Could you check a few things on this model? Use its own coordinates, in mm. A direction names the side the tool comes from. Give positions to 0.01 mm unless a question says otherwise; leave off trailing zeros. Write each loop counter-clockwise with the first axis right and the second up, starting at its lowest first coordinate (ties: lowest second). Pieces come first, ordered by that corner, then holes. Notation, with made-up numbers: (-22, -3) - (-16, -3) arc R27 ccw to (-16, 25) - close; hole circle Ø2 at (59.5, 86.5). An arc over 180 degrees is marked (long way). Answer in a Markdown table with one row per item.
from build123d import *

# Parameters (mm, degrees)
EXTRUDE_1_DEPTH          = 35
SKETCH_3_W               = 25
SKETCH_3_H               = 19
CUT_EXTRUDE_1_DEPTH      = 181.230887126
SKETCH_4_W               = 25
SKETCH_4_H               = 12.5
CUT_EXTRUDE_2_DEPTH      = 13.5
SKETCH_5_W               = 25
SKETCH_5_H               = 32
CUT_EXTRUDE_3_DEPTH      = 10
FILLET_1_R               = 3
FILLET_2_R               = 2
CUT_EXTRUDE_4_DEPTH      = 191.354670013
CUT_EXTRUDE_4_DEPTH_BACK = 191.354670013
SKETCH_6_R               = 1.5
CUT_EXTRUDE_5_DEPTH      = 189.803867534
CUT_EXTRUDE_5_DEPTH_BACK = 189.803867534
SKETCH_7_R               = 1.5
SKETCH_8_W               = 13.5
SKETCH_8_H               = 44
SKETCH_8_W_2             = 10
SKETCH_8_H_2             = 32
CUT_EXTRUDE_6_DEPTH      = 193.807936548
CUT_EXTRUDE_7_DEPTH      = 10
CUT_EXTRUDE_8_DEPTH      = 18
FILLET_3_R               = 2
SKETCH_11_W              = 10
SKETCH_11_H              = 32
EXTRUDE_2_DEPTH          = 5
CUT_EXTRUDE_10_DEPTH     = 5


with BuildPart() as part:
    # 草图1 → 凸台-拉伸1 (new body)
    with BuildSketch(Plane.XY):
        with BuildLine():
            Line((42.832374142, 47.594424801), (27.642544089, 62.784254855))
            ThreePointArc((27.642544089, 62.784254855), (27.40357385, 62.943929664), (27.121689234, 63))
            Line((27.121689234, 63), (14.544073956, 63))
            Line((14.544073956, 63), (14.544073956, 3))
            Line((14.544073956, 3), (27.121689234, 3))
            ThreePointArc((27.121689234, 3), (27.40357385, 3.056070336), (27.642544089, 3.215745145))
            Line((27.642544089, 3.215745145), (42.832374142, 18.405575199))
            ThreePointArc((42.832374142, 18.405575199), (44.044614428, 19.215568261), (45.474549341, 19.5))
            Line((45.474549341, 19.5), (159.121689234, 19.5))
            ThreePointArc((159.121689234, 19.5), (160.551624147, 19.215568261), (161.763864432, 18.405575199))
            Line((161.763864432, 18.405575199), (170.453694486, 9.715745145))
            ThreePointArc((170.453694486, 9.715745145), (170.692664725, 9.556070336), (170.974549341, 9.5))
            Line((170.974549341, 9.5), (179.738422147, 9.5))
            Line((179.738422147, 9.5), (179.738422147, 56.5))
            Line((179.738422147, 56.5), (170.974549341, 56.5))
            ThreePointArc((170.974549341, 56.5), (170.692664725, 56.443929664), (170.453694486, 56.284254855))
            Line((170.453694486, 56.284254855), (161.763864432, 47.594424801))
            ThreePointArc((161.763864432, 47.594424801), (160.551624147, 46.784431739), (159.121689234, 46.5))
            Line((159.121689234, 46.5), (45.474549341, 46.5))
            ThreePointArc((45.474549341, 46.5), (44.044614428, 46.784431739), (42.832374142, 47.594424801))
        make_face()
    extrude(amount=EXTRUDE_1_DEPTH)

    # 草图3 → 切除-拉伸1 (cut, through all)
    with BuildSketch(Plane.ZY.offset(-14.544073956)):
        with Locations((17.5, 33)):
            Rectangle(SKETCH_3_W, SKETCH_3_H)
    extrude(amount=-CUT_EXTRUDE_1_DEPTH, mode=Mode.SUBTRACT)

    # 草图4 → 切除-拉伸2 (cut)
    with BuildSketch(Plane.ZY.offset(-14.544073956)):
        with Locations((17.5, 48.75)):
            Rectangle(SKETCH_4_W, SKETCH_4_H)
        with Locations((17.5, 17.25)):
            Rectangle(SKETCH_4_W, SKETCH_4_H)
    extrude(amount=-CUT_EXTRUDE_2_DEPTH, mode=Mode.SUBTRACT)

    # 草图5 → 切除-拉伸3 (cut)
    with BuildSketch(Plane(origin=(179.738422147, 0, 0), x_dir=(0, 0, -1), z_dir=(1, 0, 0))):
        with Locations((-17.5, 33)):
            Rectangle(SKETCH_5_W, SKETCH_5_H)
    extrude(amount=-CUT_EXTRUDE_3_DEPTH, mode=Mode.SUBTRACT)

    # 圆角1
    fillet_1_edges = [part.edges().sort_by_distance(p)[0] for p in [
        (169.738422147, 23.5, 17.5),
        (169.738422147, 42.5, 17.5),
        (28.044073956, 42.5, 17.5),
        (28.044073956, 23.5, 17.5),
    ]]
    fillet(fillet_1_edges, radius=FILLET_1_R)

    # 圆角2
    fillet_2_edges = [part.edges().sort_by_distance(p)[0] for p in [
        (179.738422147, 56.5, 17.5),
        (179.738422147, 9.5, 17.5),
        (14.544073956, 3, 17.5),
        (14.544073956, 63, 17.5),
    ]]
    fillet(fillet_2_edges, radius=FILLET_2_R)

    # 草图6 → 切除-拉伸4 (cut, two sides: drawn at the far end of the back side and taken through both)
    with BuildSketch(Plane.XZ.offset(-55).offset(-CUT_EXTRUDE_4_DEPTH_BACK)):
        with Locations((23.121689234, 25)):
            Circle(SKETCH_6_R)
        with Locations((23.121689234, 10)):
            Circle(SKETCH_6_R)
    extrude(amount=CUT_EXTRUDE_4_DEPTH + CUT_EXTRUDE_4_DEPTH_BACK, mode=Mode.SUBTRACT)

    # 草图7 → 切除-拉伸5 (cut, two sides: drawn at the far end of the back side and taken through both)
    with BuildSketch(Plane.XZ.offset(-49).offset(-CUT_EXTRUDE_5_DEPTH_BACK)):
        with Locations(Location((174.974549341, 25, 0), (0, 0, 270))):
            Circle(SKETCH_7_R)
        with Locations(Location((174.974549341, 10, 0), (0, 0, 270))):
            Circle(SKETCH_7_R)
    extrude(amount=CUT_EXTRUDE_5_DEPTH + CUT_EXTRUDE_5_DEPTH_BACK, mode=Mode.SUBTRACT)

    # 草图8 → 切除-拉伸6 (cut, through all)
    with BuildSketch(Plane.XY.offset(5)):
        with Locations((21.294073956, 33)):
            Rectangle(SKETCH_8_W, SKETCH_8_H)
        with Locations((174.738422147, 33)):
            Rectangle(SKETCH_8_W_2, SKETCH_8_H_2)
    extrude(amount=-CUT_EXTRUDE_6_DEPTH, mode=Mode.SUBTRACT)

    # 草图9 → 切除-拉伸7 (cut)
    with BuildSketch(Plane(origin=(0, 0, 30), x_dir=(-1, 0, 0), z_dir=(0, 0, -1))):
        Polygon((-169.738422147, 49), (-179.738422147, 49), (-179.738422147, 17), (-169.738422147, 17), (-169.738422147, 20.5), (-169.738422147, 45.5), align=None)
    extrude(amount=-CUT_EXTRUDE_7_DEPTH, mode=Mode.SUBTRACT)

    # 草图10 → 切除-拉伸8 (cut)
    with BuildSketch(Plane.XY.offset(35)):
        with BuildLine():
            Line((169.738422147, 55.568982516), (169.738422147, 49))
            Line((169.738422147, 49), (179.738422147, 49))
            Line((179.738422147, 49), (179.738422147, 54.5))
            ThreePointArc((179.738422147, 54.5), (179.15263571, 55.914213562), (177.738422147, 56.5))
            Line((177.738422147, 56.5), (170.974549341, 56.5))
            ThreePointArc((170.974549341, 56.5), (170.692664725, 56.443929664), (170.453694486, 56.284254855))
            Line((170.453694486, 56.284254855), (169.738422147, 55.568982516))
        make_face()
    extrude(amount=-CUT_EXTRUDE_8_DEPTH, mode=Mode.SUBTRACT)

    # 圆角3
    fillet_3_edges = [part.edges().sort_by_distance(p)[0] for p in [
        (169.738422147, 55.568982516, 26),
    ]]
    fillet(fillet_3_edges, radius=FILLET_3_R)

    # 草图11 → 凸台-拉伸2 (add)
    with BuildSketch(Plane(origin=(0, 0, 0), x_dir=(-1, 0, 0), z_dir=(0, 0, -1))):
        with Locations((-174.738422147, 33)):
            Rectangle(SKETCH_11_W, SKETCH_11_H)
    extrude(amount=-EXTRUDE_2_DEPTH)

    # 草图12 → 切除-拉伸10 (cut)
    with BuildSketch(Plane(origin=(0, 0, 30), x_dir=(-1, 0, 0), z_dir=(0, 0, -1))):
        with BuildLine():
            Line((-166.738422147, 23.5), (-166.738422147, 42.5))
            ThreePointArc((-166.738422147, 42.5), (-168.859742491, 43.378679656), (-169.738422147, 45.5))
            Line((-169.738422147, 45.5), (-169.738422147, 20.5))
            ThreePointArc((-169.738422147, 20.5), (-168.859742491, 22.621320344), (-166.738422147, 23.5))
        make_face()
    extrude(amount=-CUT_EXTRUDE_10_DEPTH, mode=Mode.SUBTRACT)


solid = part.part
1) Will these pins go through, and if not, where does the flat tip stop? P1, Ø12.5, axis at x = 125, z = 18.5, coming from the +Y side; P2, Ø2, axis at x = 48.5, z = 29.5, coming from the -Y side; P3, Ø4, axis at y = 34, z = 28.5, coming from the +X side.
Check values:
| item | result |
|---|---|
| P1 | stops at y = 46.5 |
| P2 | stops at y = 19.5 |
| P3 | stops at x = 166.74 |
2) If I drill on line 1 (Y direction, x = 76, z = 21); line 2 (Z direction, x = 92.5, y = 36.5); line 3 (X direction, y = 58.25, z = 10), over which ranges is the centre line in solid material (lowest first)?
Check values:
| item | result |
|---|---|
| line 1 | y = 19.5 to 23.5, 42.5 to 46.5 |
| line 2 | z = 0 to 5, 30 to 35 |
| line 3 | x = 14.54 to 21.62, 24.62 to 32.18 |
3) Imagine slicing it at A-A (y = 39.5). List the corners of the cut face in (x, z) for me, then the cut area to 3 significant figures.
Check values:
| item | result |
|---|---|
| outline | (14.54, 30) - (166.74, 30) - (166.74, 35) - (14.54, 35) - close; (28.04, 0) - (179.74, 0) - (179.74, 5) - (28.04, 5) - close |
| area | 1,520 mm2 |
4) We'd pull the mould along Z, two halves only. Please class faces 1 (the face through (105, 33, 5)), 2 (the face through (98, 33, 0)), 3 (the face through (174, 56.5, 8)): +Z half, -Z half, draft (parallel to the pull), parting line (faces both ways), or undercut.
Check values:
| item | result |
|---|---|
| face 1 | undercut |
| face 2 | -Z half |
| face 3 | draft |
5) Imagine slicing it at C-C (z = 10). State how many separate pieces and enclosed holes the cut face has, then the cut area to 3 significant figures.
Check values:
| item | result |
|---|---|
| separate pieces | 6 |
| enclosed holes | 0 |
| area | 1,730 mm2 |
6) On a 3-axis mill with a long thin cutter (end or side, diameter ignored), from which of +Z, -Z, +X, -X, +Y, -Y can I reach the whole of each face in a straight line? I mean faces 4 (the face through (168.47, 52.6, 25.87)), 5 (the face through (166.738, 33, 32)), 6 (the face through (28.9, 22.6, 17.7)). Say none if no direction works.
Check values:
| item | result |
|---|---|
| face 4 | +Z, +Y |
| face 5 | +Z, +X |
| face 6 | -X |
7) Imagine slicing it at B-B (x = 39). List the corners of the cut face in (y, z) for me, then the cut area to 3 significant figures.
Check values:
| item | result |
|---|---|
| outline | (14.57, 0) - (51.43, 0) - (51.43, 35) - (14.57, 35) - close; hole (23.5, 5) - (42.5, 5) - (42.5, 30) - (23.5, 30) - close |
| area | 815 mm2 |
